Could you check a few things on this model? Use its own coordinates, in mm. A direction names the side the tool comes from. Coordinates: 2 decimals unless noted, no trailing zeros. Order: outer loops, then holes, each group sorted by start corner. A loop starts at its lowest first (then second) coordinate and runs counter-clockwise, first axis right, second up. Notation, with made-up numbers: (-13, 29.25) - (-7, 29.25) arc R16 ccw to (-7, 39.25) - close; hole circle Ø6 at (71.25, 57). An arc over 180 degrees is marked (long way). One line per item, written item: value.
Autodesk Inventor part; units mm, degrees
ref_plane "作業平面1" through (-10, -13, 5) normal (-1, 0, 0) x (0, 0, 1)
ref_plane "YZ Plane" through (0, 0, 0) normal (1, 0, 0) x (0, 1, 0)
ref_plane "XZ Plane" through (0, 0, 0) normal (0, 1, 0) x (-1, 0, 0)
sketch "スケッチ1" plane through (0, 0, 0) normal (0, 1, 0) x (-1, 0, 0)
  line L0 (0, 0) -> (0, -30)
  circle A0 centre (0, 0) radius 3.05
  circle A1 centre (0, -30) radius 3.05
  circle A2 centre (0, 0) radius 5
  circle A3 centre (0, -30) radius 5
  line L1 (5, 0) -> (5, -30)
  line L2 (0, -5) -> (5, -5)
  line L3 (0, -25) -> (5, -25)
  line L4 (0, 5) -> (5, 5)
  line L5 (5, 5) -> (5, 0)
  line L6 (0, -35) -> (5, -35)
  line L7 (5, -35) -> (5, -30)
  line L8 (5, 5) -> (10, 5)
  line L9 (10, 5) -> (10, -35)
  line L10 (10, -35) -> (5, -35)
  line L11 (5, -35) -> (5, 5)
  dimension "d0" = 30
  dimension "d1" = 6.1
  dimension "d2" = 6.1
  dimension "d3" = 10
  dimension "d4" = 10
  dimension "d5" = 5
  dimension "d6" = 40
extrude "押し出し1" add sketch "スケッチ1" along normal blind 50 contours A2 | A2 L1 L2 | L3 L1 A3 | A3 | L4 L5 A2 | L5 L8 L9 L10 L7 L1 | L7 L6 A3
sketch "スケッチ2" plane through (0, 50, 0) normal (0, 1, 0) x (1, 0, 0)
  line L0 (-10, 35) -> (-10, -5)
  line L1 (0, 35) -> (-10, 35)
  line L2 (-10, -5) -> (-5, -5)
  line L3 (-5, -5) -> (-5, 35)
  line L4 (-5, 35) -> (-10, 35)
  line L5 (-10, 35) -> (-10, -5)
  point P0 (0, 0)
extrude "押し出し2" add sketch "スケッチ2" along normal blind 15
sketch "スケッチ3" plane through (0, 0, 0) normal (0, -1, 0) x (1, 0, 0)
  line L0 (-10, 5) -> (0, 5)
  line L1 (-5, -35) -> (-5, -25)
  line L2 (-10, 5) -> (-5, 5)
  line L3 (-5, 5) -> (-5, -35)
  line L4 (-5, -35) -> (-10, -35)
  line L5 (-10, -35) -> (-10, 5)
  point P0 (0, 0)
extrude "押し出し3" add sketch "スケッチ3" along normal blind 15
sketch "スケッチ4" plane through (-5, 0, -25) normal (1, 0, 0) x (0, 0, -1)
  circle A0 centre (-15, 25) radius 7
  line L0 (-30, 0) -> (-30, 50)
  line L1 (-20, 0) -> (-30, 0)
  point P0 (-25, 0)
  dimension "d13" = 14
  dimension "d14" = 15
  dimension "d15" = 25
extrude "押し出し4" cut sketch "スケッチ4" along normal blind 50
sketch "スケッチ5" plane through (0, 0, -35) normal (0, 0, -1) x (-1, 0, 0)
  line L0 (10, -15) -> (10, 65)
  line L1 (10, 65) -> (5, 65)
  line L2 (10, -15) -> (5, -15)
  line L3 (5, -15) -> (5, 65)
  line L4 (5, 65) -> (10, 65)
  line L5 (10, 65) -> (10, -15)
  point P0 (0, 0)
extrude "押し出し5" add sketch "スケッチ5" along normal blind 20
ref_plane "作業平面1" through (-10, -13, 5) normal (-1, 0, 0) x (0, 0, 1)
sketch "スケッチ6" plane through (-10, -13, 5) normal (-1, 0, 0) x (0, 0, 1)
  line L0 (0, -2) -> (0, 78)
  line L1 (0, 78) -> (-60, 78)
  line L2 (-60, -2) -> (-60, 78)
  line L3 (0, -2) -> (-60, -2)
  point P0 (-5, 13)
extrude "押し出し6" add sketch "スケッチ6" along normal blind 5
sketch "スケッチ7" plane through (-5, 0, 5) normal (0, 0, 1) x (1, 0, 0)
  line L0 (-10, 63) -> (-10, -13)
  line L1 (-10, 25) -> (-132.5, 25)
  circle A0 centre (-132.5, 25) radius 122.5
  line L2 (-10, 65) -> (-16.7146, 65)
  line L3 (0, -15) -> (-10, -15)
  line L4 (-10, -15) -> (-16.7146, -15)
  line L5 (0, 0) -> (5, 0)
  line L6 (5, 0) -> (5, 50)
  line L7 (0, 50) -> (5, 50)
  line L8 (0, 50) -> (0, 65)
  line L9 (0, 65) -> (-10, 65)
  line L10 (-10, -15) -> (-10, 65)
  line L11 (0, -15) -> (-10, -15)
  line L12 (0, 0) -> (0, -15)
  dimension "d23" = 122.5
  dimension "d24" = 180
extrude "押し出し7" add sketch "スケッチ7" against normal blind 60 contours L0 A0 L2 L10 | L0 L10 L4 A0
properties part number "hand2_13" material "ABS プラスチック"
Item 1: I want a section at C-C on y = 22.5. Please give me the cut outline in (x, z).
Conclusion:
outline: (-15.03, -55) - (-5, -55) - (-5, -35) - (0, -35) arc R5 ccw to (0, -25) - (-5, -25) - (-5, -3.46) - (3.61, -3.46) arc R5 ccw to (0, 5) - (-15.03, 5) - close; hole circle Ø6.1 at (0, -30); hole circle Ø6.1 at (0, 0)
Item 2: Thinking about a two-plate mould opening in Y: for faces 4 (the face through (-3.3, 0, 0.1)), 5 (the face through (-11, 24, 5)), 6 (the face through (-15, 24.4, -24.6)), which applies, pulls with the +Y half, pulls with the -Y half, needs draft (parallel to the pull), parting line crosses it, or undercut?
Conclusion:
face 4: pulls with the -Y half
face 5: needs draft
face 6: undercut
Item 3: I want a section at A-A on x = -20. Please give me the cut outline in (y, z), then the cut area to 3 significant figures.
Conclusion:
outline: (-15, -55) - (-9.64, -55) - (-9.64, 5) - (-15, 5) - close; (59.64, -55) - (65, -55) - (65, 5) - (59.64, 5) - close
area: 643 mm²
Item 4: For faces 1 (the face through (-2, 25, -25)), 2 (the face through (-2, 25, -35)), 3 (the face through (-3.3, 0, -29.9)), which set-ups out of +Z, -Z, +X, -X, +Y, -Y let a thin tool reach every point of the face, with its end or its side?
Conclusion:
face 1: +X, +Y, -Y
face 2: -Z, +X, +Y, -Y
face 3: +Z, -Z, +X, -Y
Item 5: I'm going to push flat-ended pins straight in: pin 1 Ø11 at (x, z) = (2.5, -28.5) entering from -Y; pin 2 Ø6 at (y, z) = (38.5, -45) entering from -X; pin 3 Ø2 at (x, z) = (-2.5, -28) entering from +Y; pin 4 Ø12 at (x, z) = (0, -22) entering from +Y. Where does each tip first touch, or does it pass through?
Conclusion:
pin 1: y = 0
pin 2: x = -16.12
pin 3: y = 50
pin 4: y = 65
Item 6: I want a section at D-D on z = -48.5. Please give me the cut outline in (x, y), then the cut area to 3 significant figures.
Conclusion:
outline: (-21.71, -15) - (-5, -15) - (-5, 65) - (-21.71, 65) arc R122.5 cw to start
area: 977 mm²
Item 7: If I drill on probe 1 along Z at (x, y) = (0, 13); probe 2 along Z at (x, y) = (2, 21.5); probe 3 along X at (y, z) = (26.5, -30), over which ranges is the centre line in solid material (lowest first)?
Conclusion:
probe 1: -35 to -33.05, -26.95 to -25, -5 to -3.05, 3.05 to 5
probe 2: -34.58 to -32.3, -27.7 to -25.42, -3.94 to -2.3, 2.3 to 4.58
probe 3: -15.01 to -3.05, 3.05 to 5
Item 8: I want a section at B-B on z = -29. Please give me the cut outline in (x, y).
Conclusion:
outline: (-21.71, -15) - (-5, -15) - (-5, 0) - (-2.88, 0) - (-2.88, 50) - (-5, 50) - (-5, 65) - (-21.71, 65) arc R122.5 cw to start; (2.88, 0) - (4.9, 0) - (4.9, 50) - (2.88, 50) - close
